from build123d import *

# Parameters (mm, degrees)
F0_W     = 127
F0_H     = 127
F1_DEPTH = 2.54
F2_R     = 5.08
F3_W     = 20.884663
F3_H     = 43.656439
F4_DEPTH = 25.4


with BuildPart() as f1:
    # F0 (on Top) → F1 (new body)
    with BuildSketch(Plane.XY):
        Rectangle(F0_W, F0_H)
    extrude(amount=F1_DEPTH)

    # F2
    f2_edges = [f1.edges().sort_by_distance(p)[0] for p in [
        (63.5, -63.5, 1.27),
        (63.5, 63.5, 1.27),
        (-63.5, 63.5, 1.27),
        (-63.5, -63.5, 1.27),
    ]]
    fillet(f2_edges, radius=F2_R)

    # F3 (on face) → F4 (cut)
    with BuildSketch(Plane.XY.offset(2.54)):
        with Locations((-33.551299, -4.489437)):
            Rectangle(F3_W, F3_H)
    extrude(amount=-F4_DEPTH, mode=Mode.SUBTRACT)


solid = f1.part
Geometry check sheet. Reference: the model listing, model coordinates, mm. Give positions to 0.01 mm unless a question says otherwise; leave off trailing zeros. Order: outer loops, then holes, each group sorted by start corner. A loop starts at its lowest first (then second) coordinate and runs counter-clockwise, first axis right, second up. Notation, with made-up numbers: M 8.5,33 L 45.5,33 A25 ccw 45.5,45 Z; hole C 47,15.25 d7. An arc over 180 degrees is marked long. Use a Markdown table: item, result.
Item 1: Section check B-B (z = 0.7). Record the cut outline in (x, y), and give its area (3 significant figures).
Answers follow:
| item | result |
|---|---|
| outline | M -63.5,-58.42 A5.08 ccw -58.42,-63.5 L 58.42,-63.5 A5.08 ccw 63.5,-58.42 L 63.5,58.42 A5.08 ccw 58.42,63.5 L -58.42,63.5 A5.08 ccw -63.5,58.42 Z; hole M -43.99,-26.32 L -23.11,-26.32 L -23.11,17.34 L -43.99,17.34 Z |
| area | 15,200 mm2 |
Item 2: Section check A-A (y = 5). Record the cut outline in (x, z).
Answers follow:
| item | result |
|---|---|
| outline | M -63.5,0 L -43.99,0 L -43.99,2.54 L -63.5,2.54 Z; M -23.11,0 L 63.5,0 L 63.5,2.54 L -23.11,2.54 Z |
Item 3: Material ranges on line 1 along Y through (x, z) = (-26.5, 1.45); line 2 along X through (y, z) = (-10.5, 0.7); line 3 along Y through (x, z) = (58.5, 1.7), recorded low to high.
Answers follow:
| item | result |
|---|---|
| line 1 | y = -63.5 to -26.32, 17.34 to 63.5 |
| line 2 | x = -63.5 to -43.99, -23.11 to 63.5 |
| line 3 | y = -63.5 to 63.5 |
